from build123d import *

# Parameters (mm, degrees)
SKETCH1_R           = 19.05
SKETCH1_R_2         = 2.794
BOSS_EXTRUDE1_DEPTH = 2.54
SKETCH2_R           = 19.05
BOSS_EXTRUDE2_DEPTH = 6.35
SKETCH3_R           = 5.08
CUT_EXTRUDE1_DEPTH  = 3.81
FILLET1_R           = 3.81
FILLET2_R           = 1.27


with BuildPart() as part:
    # Sketch1 → Boss-Extrude1 (new body)
    with BuildSketch(Plane(origin=(0, 0, 0), x_dir=(1, 0, 0), z_dir=(0, 1, 0))):
        with Locations(Location((0, 0, 0), (0, 0, 270))):
            Circle(SKETCH1_R)
        with Locations(Location((0, 0, 0), (0, 0, 270))):
            Circle(SKETCH1_R_2, mode=Mode.SUBTRACT)
    extrude(amount=BOSS_EXTRUDE1_DEPTH)

    # Sketch2 → Boss-Extrude2 (add)
    with BuildSketch(Plane(origin=(0, 2.54, 0), x_dir=(1, 0, 0), z_dir=(0, 1, 0))):
        with Locations(Location((0, 0, 0), (0, 0, 270))):
            Circle(SKETCH2_R)
        Polygon((5.42593783, 0), (2.712968915, 4.699), (-2.712968915, 4.699), (-5.42593783, 0), (-2.712968915, -4.699), (2.712968915, -4.699), align=None, mode=Mode.SUBTRACT)
    extrude(amount=BOSS_EXTRUDE2_DEPTH)

    # Sketch3 → Cut-Extrude1 (cut)
    with BuildSketch(Plane(origin=(0, 8.89, 0), x_dir=(1, 0, 0), z_dir=(0, 1, 0))):
        with Locations(Location((0, 12.065, 0), (0, 0, 270))):
            Circle(SKETCH3_R)
        with Locations(Location((0, -12.065, 0), (0, 0, 270))):
            Circle(SKETCH3_R)
    extrude(amount=-CUT_EXTRUDE1_DEPTH, mode=Mode.SUBTRACT)

    # Fillet1
    fillet1_edges = [part.edges().sort_by_distance(p)[0] for p in [
        (0, 5.08, -17.145),
        (0, 5.08, 6.985),
    ]]
    fillet(fillet1_edges, radius=FILLET1_R - 0.0001)  # a hair under: the kernel refuses the full size

    # Fillet2
    fillet2_edges = [part.edges().sort_by_distance(p)[0] for p in [
        (0, 0, -19.05),
    ]]
    fillet(fillet2_edges, radius=FILLET2_R)


solid = part.part
CAD build for the part. Positions are in the model's coordinates, mm. A direction names the side the tool comes from. Give positions to 0.01 mm unless a question says otherwise; leave off trailing zeros. Order: outer loops, then holes, each group sorted by start corner. A loop starts at its lowest first (then second) coordinate and runs counter-clockwise, first axis right, second up. Notation, with made-up numbers: (38, 64.25) -> (80, 64.25) arc R16 ccw to (80, 80.25) -> close; hole circle Ø2 at (-37, -25.5). An arc over 180 degrees is marked (long way). Return JSON: item names as keys, results as strings.
Q1. Flat gauge pins, fed straight in: pin 1 (5 mm diameter, centred on y = 3.5, z = -1.5, fed in from +X); pin 2 (1.6 mm diameter, centred on x = 1, y = 4.5, fed in from -Z); pin 3 (5 mm diameter, centred on x = -8, y = 5, fed in from +Z). Where does each tip first touch, or does it go through?
Working result:
{"pin 1": "x = 19.05", "pin 2": "z = -19.05", "pin 3": "z = 18.24"}
Q2. Mould opens along X. For faces 3 (the face through (-2.3, 2.54, -2.2)), 4 (the face through (-4, 8.89, 4)), 5 (the face through (-11.59, 5.03, -15.12)) say: pulls with the +X half, pulls with the -X half, needs draft (parallel to the pull), parting line crosses it, or undercut.
Working result:
{"face 3": "undercut", "face 4": "needs draft", "face 5": "parting line crosses it"}
Q3. Drill centre lines: line 1 (Z direction, x = 0.5, y = 8.75); line 2 (X direction, y = 4.25, z = -3); line 3 (X direction, y = 0.8, z = 0). Where is each one in solid material? Low to high.
Working result:
{"line 1": "-19.04 to -17.12, -7.01 to -4.7, 4.7 to 7.01, 17.12 to 19.04", "line 2": "-18.81 to -3.69, 3.69 to 18.81", "line 3": "-18.96 to -2.79, 2.79 to 18.96"}
Q4. Saw through at A-A (y = 4.5). Write the cut outline in (x, z).
Working result:
{"outline": "circle Ø38.1 at (0, 0); hole (-5.43, 0) -> (-2.71, -4.7) -> (2.71, -4.7) -> (5.43, 0) -> (2.71, 4.7) -> (-2.71, 4.7) -> close"}
Q5. Saw through at B-B (y = 6.75). Count the separate pieces of the cut face and the enclosed holes in it, then the cut area to 3 significant figures.
Working result:
{"separate pieces": "1", "enclosed holes": "3", "area": "941 mm²"}
Q6. Which spindle directions (+Z, -Z, +X, -X, +Y, -Y) get a long thin tool onto all of the face, cutting with end or side? Do faces 1 (the face through (0, 6, -4.699)), 2 (the face through (-2.728, 1.252, -0.606)). Say none if no direction does.
Working result:
{"face 1": "+Y", "face 2": "+Y, -Y"}
